Part model, mm, in its own coordinate system. A direction names the side the tool comes from. Round coordinates to 2 decimals unless told otherwise and drop trailing zeros. Loops run counter-clockwise (first coordinate to the right, second up) from the corner with the lowest first, then second, coordinate; pieces in that order, holes last. Notation, with made-up numbers: M 35,41.25 L 91,41.25 A22 cw 91,78.25 Z; hole C -31.5,-25 d1. An arc over 180 degrees is marked long. Write each question's results on one line, items separated by ' | '.
from build123d import *

# Parameters (mm, degrees)
CROQUIS1_W              = 161
CROQUIS1_H              = 51.5812
SALIENTE_EXTRUIR1_DEPTH = 3
CORTAR_EXTRUIR1_REACH   = 5
CROQUIS2_R              = 1.5
CROQUIS2_R_2            = 4
CORTAR_EXTRUIR2_REACH   = 5
CROQUIS3_R              = 1.5
CORTAR_EXTRUIR3_REACH   = 53.581
CORTAR_EXTRUIR4_REACH   = 5
CORTAR_EXTRUIR5_REACH   = 5
CORTAR_EXTRUIR6_REACH   = 5
CORTAR_EXTRUIR7_REACH   = 5
CORTAR_EXTRUIR8_REACH   = 5
CROQUIS9_R              = 1.5


with BuildPart() as part:
    # Croquis1 → Saliente-Extruir1 (new body)
    with BuildSketch(Plane(origin=(0, 0, 0), x_dir=(0, 0, -1), z_dir=(1, 0, 0))):
        Rectangle(CROQUIS1_W, CROQUIS1_H)
    extrude(amount=SALIENTE_EXTRUIR1_DEPTH)

    # Croquis2 → Cortar-Extruir1 (cut, up to next)
    with BuildSketch(Plane(origin=(3, 0, 0), x_dir=(0, 0, -1), z_dir=(1, 0, 0)), mode=Mode.PRIVATE) as cortar_extruir1_sk1:
        with Locations((-75.5, 20.7906)):
            Circle(CROQUIS2_R)
    cortar_extruir1_tool1 = extrude(cortar_extruir1_sk1.sketch, amount=-CORTAR_EXTRUIR1_REACH, mode=Mode.PRIVATE) & part.part
    add(cortar_extruir1_tool1.solids().sort_by_distance((3, 20.7906, 75.5))[0], mode=Mode.SUBTRACT)
    # Croquis2 → Cortar-Extruir1 (cut, up to next)
    with BuildSketch(Plane(origin=(3, 0, 0), x_dir=(0, 0, -1), z_dir=(1, 0, 0)), mode=Mode.PRIVATE) as cortar_extruir1_sk2:
        with Locations((-1.88, 20.7906)):
            Circle(CROQUIS2_R)
    cortar_extruir1_tool2 = extrude(cortar_extruir1_sk2.sketch, amount=-CORTAR_EXTRUIR1_REACH, mode=Mode.PRIVATE) & part.part
    add(cortar_extruir1_tool2.solids().sort_by_distance((3, 20.7906, 1.88))[0], mode=Mode.SUBTRACT)
    # Croquis2 → Cortar-Extruir1 (cut, up to next)
    with BuildSketch(Plane(origin=(3, 0, 0), x_dir=(0, 0, -1), z_dir=(1, 0, 0)), mode=Mode.PRIVATE) as cortar_extruir1_sk3:
        with Locations((-51.5, -3.2094)):
            Circle(CROQUIS2_R_2)
    cortar_extruir1_tool3 = extrude(cortar_extruir1_sk3.sketch, amount=-CORTAR_EXTRUIR1_REACH, mode=Mode.PRIVATE) & part.part
    add(cortar_extruir1_tool3.solids().sort_by_distance((3, -3.2094, 51.5))[0], mode=Mode.SUBTRACT)

    # Croquis3 → Cortar-Extruir2 (cut, up to next)
    with BuildSketch(Plane.ZY, mode=Mode.PRIVATE) as cortar_extruir2_sk1:
        with Locations((-35.801477372, -16.2094)):
            Circle(CROQUIS3_R)
    cortar_extruir2_tool1 = extrude(cortar_extruir2_sk1.sketch, amount=-CORTAR_EXTRUIR2_REACH, mode=Mode.PRIVATE) & part.part
    add(cortar_extruir2_tool1.solids().sort_by_distance((0, -16.2094, -35.801477))[0], mode=Mode.SUBTRACT)

    # Croquis4 → Cortar-Extruir3 (cut, up to next)
    with BuildSketch(Plane(origin=(0, 25.7906, 0), x_dir=(1, 0, 0), z_dir=(0, 1, 0)), mode=Mode.PRIVATE) as cortar_extruir3_sk1:
        Polygon((3, 80.5), (0, 80.5), (0, 72.980420108), (3, 66.546899347), align=None)
    cortar_extruir3_tool1 = extrude(cortar_extruir3_sk1.sketch, amount=-CORTAR_EXTRUIR3_REACH, mode=Mode.PRIVATE) & part.part
    add(cortar_extruir3_tool1.solids().sort_by_distance((1.649807, 25.7906, -74.971199))[0], mode=Mode.SUBTRACT)

    # Croquis5 → Cortar-Extruir4 (cut, up to next)
    with BuildSketch(Plane.ZY, mode=Mode.PRIVATE) as cortar_extruir4_sk1:
        Polygon((-72.980420108, -25.7906), (-72.980420108, -21.149469815), (-55.595458212, -21.2094), (3.759789946, -25.7906), align=None)
    cortar_extruir4_tool1 = extrude(cortar_extruir4_sk1.sketch, amount=-CORTAR_EXTRUIR4_REACH, mode=Mode.PRIVATE) & part.part
    add(cortar_extruir4_tool1.solids().sort_by_distance((0, -23.974753, -46.380283))[0], mode=Mode.SUBTRACT)

    # Croquis6 → Cortar-Extruir5 (cut, up to next)
    with BuildSketch(Plane.ZY, mode=Mode.PRIVATE) as cortar_extruir5_sk1:
        Polygon((-72.980420108, 25.7906), (-72.980420108, 2.2906), (-52.770420108, 14.0406), (-52.770420108, 25.7906), align=None)
    cortar_extruir5_tool1 = extrude(cortar_extruir5_sk1.sketch, amount=-CORTAR_EXTRUIR5_REACH, mode=Mode.PRIVATE) & part.part
    add(cortar_extruir5_tool1.solids().sort_by_distance((0, 16.651711, -63.998198))[0], mode=Mode.SUBTRACT)

    # Croquis7 → Cortar-Extruir6 (cut, up to next)
    with BuildSketch(Plane.ZY, mode=Mode.PRIVATE) as cortar_extruir6_sk1:
        Polygon((-52.770420108, 25.7906), (-41.670420108, 25.7906), (-52.770420108, 14.0406), align=None)
    cortar_extruir6_tool1 = extrude(cortar_extruir6_sk1.sketch, amount=-CORTAR_EXTRUIR6_REACH, mode=Mode.PRIVATE) & part.part
    add(cortar_extruir6_tool1.solids().sort_by_distance((0, 21.873933, -49.07042))[0], mode=Mode.SUBTRACT)

    # Croquis8 → Cortar-Extruir7 (cut, up to next)
    with BuildSketch(Plane.ZY, mode=Mode.PRIVATE) as cortar_extruir7_sk1:
        Polygon((8.660254038, 0), (4.330127019, 7.5), (-4.330127019, 7.5), (-8.660254038, 0), (-4.330127019, -7.5), (4.330127019, -7.5), align=None)
    cortar_extruir7_tool1 = extrude(cortar_extruir7_sk1.sketch, amount=-CORTAR_EXTRUIR7_REACH, mode=Mode.PRIVATE) & part.part
    add(cortar_extruir7_tool1.solids().sort_by_distance((0, 0, 0))[0], mode=Mode.SUBTRACT)
    # Croquis8 → Cortar-Extruir7 (cut, up to next)
    with BuildSketch(Plane.ZY, mode=Mode.PRIVATE) as cortar_extruir7_sk2:
        Polygon((25.604154883, 9.319150251), (22.099721379, 12.259719112), (17.800897292, 10.695075102), (17.006506709, 6.189862231), (20.510940213, 3.24929337), (24.8097643, 4.81393738), align=None)
    cortar_extruir7_tool2 = extrude(cortar_extruir7_sk2.sketch, amount=-CORTAR_EXTRUIR7_REACH, mode=Mode.PRIVATE) & part.part
    add(cortar_extruir7_tool2.solids().sort_by_distance((0, 7.754506, 21.305331))[0], mode=Mode.SUBTRACT)
    # Croquis8 → Cortar-Extruir7 (cut, up to next)
    with BuildSketch(Plane.ZY, mode=Mode.PRIVATE) as cortar_extruir7_sk3:
        Polygon((-23.988727728, -11.985830273), (-19.711232592, -14.811812276), (-15.125112818, -12.520383825), (-14.816488181, -7.402973371), (-19.093983317, -4.576991368), (-23.68010309, -6.868419819), align=None)
    cortar_extruir7_tool3 = extrude(cortar_extruir7_sk3.sketch, amount=-CORTAR_EXTRUIR7_REACH, mode=Mode.PRIVATE) & part.part
    add(cortar_extruir7_tool3.solids().sort_by_distance((0, -9.694402, -19.402608))[0], mode=Mode.SUBTRACT)
    # Croquis8 → Cortar-Extruir7 (cut, up to next)
    with BuildSketch(Plane.ZY, mode=Mode.PRIVATE) as cortar_extruir7_sk4:
        Polygon((-22.123245507, 9.737186974), (-21.644369238, 5.360424201), (-17.614543355, 3.58676183), (-14.063593742, 6.189862231), (-14.542470011, 10.566625004), (-18.572295894, 12.340287376), align=None)
    cortar_extruir7_tool4 = extrude(cortar_extruir7_sk4.sketch, amount=-CORTAR_EXTRUIR7_REACH, mode=Mode.PRIVATE) & part.part
    add(cortar_extruir7_tool4.solids().sort_by_distance((0, 7.963525, -18.09342))[0], mode=Mode.SUBTRACT)
    # Croquis8 → Cortar-Extruir7 (cut, up to next)
    with BuildSketch(Plane.ZY, mode=Mode.PRIVATE) as cortar_extruir7_sk5:
        Polygon((26.752701341, -9.737186974), (25.898994771, -4.895576423), (21.279183753, -3.214102725), (17.513079305, -6.374239578), (18.366785876, -11.215850129), (22.986596894, -12.897323827), align=None)
    cortar_extruir7_tool5 = extrude(cortar_extruir7_sk5.sketch, amount=-CORTAR_EXTRUIR7_REACH, mode=Mode.PRIVATE) & part.part
    add(cortar_extruir7_tool5.solids().sort_by_distance((0, -8.055713, 22.13289))[0], mode=Mode.SUBTRACT)
    # Croquis8 → Cortar-Extruir7 (cut, up to next)
    with BuildSketch(Plane.ZY, mode=Mode.PRIVATE) as cortar_extruir7_sk6:
        Polygon((-50.300771297, 0), (-46.052967767, -7.357411534), (-37.557360708, -7.357411534), (-33.309557178, 0), (-37.557360708, 7.357411534), (-46.052967767, 7.357411534), align=None)
    cortar_extruir7_tool6 = extrude(cortar_extruir7_sk6.sketch, amount=-CORTAR_EXTRUIR7_REACH, mode=Mode.PRIVATE) & part.part
    add(cortar_extruir7_tool6.solids().sort_by_distance((0, 0, -41.805164))[0], mode=Mode.SUBTRACT)
    # Croquis8 → Cortar-Extruir7 (cut, up to next)
    with BuildSketch(Plane.ZY, mode=Mode.PRIVATE) as cortar_extruir7_sk7:
        Polygon((37.746685044, 13.738669798), (41.711835056, 10.411513886), (46.575811604, 12.18185657), (47.474638141, 17.279355166), (43.509488129, 20.606511078), (38.645511581, 18.836168394), align=None)
    cortar_extruir7_tool7 = extrude(cortar_extruir7_sk7.sketch, amount=-CORTAR_EXTRUIR7_REACH, mode=Mode.PRIVATE) & part.part
    add(cortar_extruir7_tool7.solids().sort_by_distance((0, 15.509012, 42.610662))[0], mode=Mode.SUBTRACT)
    # Croquis8 → Cortar-Extruir7 (cut, up to next)
    with BuildSketch(Plane.ZY, mode=Mode.PRIVATE) as cortar_extruir7_sk8:
        Polygon((38.645511581, -14.065815903), (39.684095326, -19.955917015), (45.304364392, -22.001527663), (49.886049713, -18.157037201), (48.847465968, -12.266936089), (43.227196902, -10.221325441), align=None)
    cortar_extruir7_tool8 = extrude(cortar_extruir7_sk8.sketch, amount=-CORTAR_EXTRUIR7_REACH, mode=Mode.PRIVATE) & part.part
    add(cortar_extruir7_tool8.solids().sort_by_distance((0, -16.111427, 44.265781))[0], mode=Mode.SUBTRACT)

    # Croquis9 → Cortar-Extruir8 (cut, up to next)
    with BuildSketch(Plane.ZY, mode=Mode.PRIVATE) as cortar_extruir8_sk1:
        with Locations((-35.801477372, 20.7906)):
            Circle(CROQUIS9_R)
    cortar_extruir8_tool1 = extrude(cortar_extruir8_sk1.sketch, amount=-CORTAR_EXTRUIR8_REACH, mode=Mode.PRIVATE) & part.part
    add(cortar_extruir8_tool1.solids().sort_by_distance((0, 20.7906, -35.801477))[0], mode=Mode.SUBTRACT)


solid = part.part
Item 1: Wall check: L1, parallel to Y at x = 2.15, z = 75.5; L2, parallel to Z at x = 1.65, y = -1; L3, parallel to Z at x = 1.65, y = 1.5. Give the ranges that are in metal, low to high.
Filled sheet:
L1: -25.79 to 19.29, 22.29 to 25.79 | L2: -69.44 to -49.72, -33.89 to -8.08, 8.08 to 48.17, 54.83 to 80.5 | L3: -69.44 to -49.43, -34.18 to -7.79, 7.79 to 80.5
Item 2: Band-saw the part on C-C on z = 75.5. Give the cut face in (x, y), and give its area (3 significant figures).
Filled sheet:
outline: M 0,-25.79 L 3,-25.79 L 3,19.29 L 0,19.29 Z; M 0,22.29 L 3,22.29 L 3,25.79 L 0,25.79 Z | area: 146 mm^2
Item 3: Two-plate mould, pull along Z, no slides. Class faces 3 (the flat face through (1.48, 4.02, 22.63)), 4 (the flat face through (3, -5, 8)): +Z half, -Z half, draft (parallel to the pull), parting line (faces both ways), or undercut.
Filled sheet:
face 3: undercut | face 4: draft
Item 4: Band-saw the part on A-A on z = 51.5. Give the cut face in (x, y).
Filled sheet:
outline: M 0,-25.79 L 3,-25.79 L 3,-7.21 L 0,-7.21 Z; M 0,0.79 L 3,0.79 L 3,25.79 L 0,25.79 Z
Item 5: Drop a flat-ended pin along its axis: P1, Ø2.5, axis at y = 20.79, z = -35.8, coming from the -X side. Give the stop position or say it passes through.
Filled sheet:
P1: through
Item 6: Band-saw the part on D-D on x = 1. Count the separate pieces of the cut face and the enclosed holes in it, and give its area (3 significant figures).
Filled sheet:
separate pieces: 1 | enclosed holes: 13 | area: 6,370 mm^2
Item 7: Which spindle directions (+Z, -Z, +X, -X, +Y, -Y) get a long thin tool onto all of the face, cutting with end or side? Do faces 1 (the flat face through (1.48, -11.34, 24.84)), 2 (the flat face through (1, 25.791, 20)). Say none if no direction does.
Filled sheet:
face 1: +X, -X | face 2: +Z, -Z, +X, -X, +Y
Item 8: Band-saw the part on B-B on z = 1.88. Give the cut face in (x, y), and give its area (3 significant figures).
Filled sheet:
outline: M 0,-25.65 L 3,-25.65 L 3,-7.5 L 0,-7.5 Z; M 0,7.5 L 3,7.5 L 3,19.29 L 0,19.29 Z; M 0,22.29 L 3,22.29 L 3,25.79 L 0,25.79 Z | area: 100 mm^2
